```python
from build123d import *

# Parameters (mm, degrees)
CUT_EXTRUDE_START   = 10
CUT_EXTRUDE_1_DEPTH = 112.622366364


with BuildPart() as part:
    # Эскиз1 → Повернуть1 (revolve)
    with BuildSketch(Plane.XY):
        Polygon((0, 0), (0, 12.5), (15, 12.5), (15, 14), (55, 14), (55, 12.5), (70, 12.5), (70, 11), (120, 11), (120, 0), align=None)
    revolve(axis=Axis((120, 0, 0), (-1, 0, 0)))

    # Эскиз3 → Вырез-Вытянуть1 (cut, through all)
    with BuildSketch(Plane(origin=(0, 0, 0), x_dir=(1, 0, 0), z_dir=(0, 1, 0)).offset(CUT_EXTRUDE_START)):
        with BuildLine():
            Line((21, 4), (49, 4))
            ThreePointArc((49, 4), (53, 0), (49, -4))
            Line((49, -4), (21, -4))
            ThreePointArc((21, -4), (17, 0), (21, 4))
        make_face()
    extrude(amount=CUT_EXTRUDE_1_DEPTH, mode=Mode.SUBTRACT)


solid = part.part
```
Verification items for the finished model (mm, model axes). A direction names the side the tool comes from. Round coordinates to 2 decimals unless told otherwise and drop trailing zeros. Write each loop counter-clockwise with the first axis right and the second up, starting at its lowest first coordinate (ties: lowest second). Pieces come first, ordered by that corner, then holes.
1. Section check B-B on z = -1.25. Enter the section's corners in (x, y).
2. Gauge pin test, flat ends, axial feed: P1, Ø12, axis at x = 34.5, y = -8.5, coming from the -Z side (3 decimals); P2, Ø2, axis at x = 60.5, z = -2, coming from the -Y side; P3, Ø5, axis at y = 6.5, z = 2.5, coming from the -X side; P4, Ø2, axis at x = 40.5, y = 7.5, coming from the -Z side. Record the tip position at first contact, or that the pin passes through.
3. Section check D-D on y = -7.75. Enter the section's corners in (x, z).
4. Scan lines: L1, parallel to X at y = 9, z = 7; L2, parallel to Z at x = 46.5, y = 0.5; L3, parallel to Y at x = 53.5, z = -4.25. Record each from-to range of solid material in increasing order.
5. Section check C-C on x = 86. Enter the section's corners in (y, z), plus the area to 3 significant figures.
6. Access from +Z, -Z, +X, -X, +Y, -Y to the whole of each face (thin tool, end or side, straight path). Record for faces 4 (the cylindrical face through (62.605, 11.923, -3.755)), 5 (the flat face through (15, 5.3, -11.5)), 6 (the flat face through (35, 12, 4)).
7. Draft check along Z on faces 1 (the cylindrical face through (35.28, 12.932, 5.362)), 2 (the cylindrical face through (53, 12, 0)), 3 (the flat face through (70, 5, 10)). Enter one of: +Z half, -Z half, draft (parallel to the pull), parting line (faces both ways), or undercut.
8. Section check A-A on y = 0. Enter the section's corners in (x, z), plus the area to 3 significant figures.
Answer:
1. outline: (0, -12.44) - (15, -12.44) - (15, -13.94) - (55, -13.94) - (55, -12.44) - (70, -12.44) - (70, -10.93) - (120, -10.93) - (120, 10.93) - (70, 10.93) - (70, 12.44) - (55, 12.44) - (55, 13.94) - (52.8, 13.94) - (52.8, 10) - (17.2, 10) - (17.2, 13.94) - (15, 13.94) - (15, 12.44) - (0, 12.44) - close
2. P1: stops at z = -13.775
2. P2: stops at y = -12.46
2. P3: stops at x = 0
2. P4: stops at z = -12.4
3. outline: (0, -9.81) - (15, -9.81) - (15, -11.66) - (55, -11.66) - (55, -9.81) - (70, -9.81) - (70, -7.81) - (120, -7.81) - (120, 7.81) - (70, 7.81) - (70, 9.81) - (55, 9.81) - (55, 11.66) - (15, 11.66) - (15, 9.81) - (0, 9.81) - close
4. L1: x = 0 to 70
4. L2: z = -13.99 to 13.99
4. L3: y = -13.34 to 13.34
5. outline: circle Ø22 at (0, 0)
5. area: 380 mm2
6. face 4: +X
6. face 5: -X
6. face 6: +Y
7. face 1: parting line
7. face 2: undercut
7. face 3: draft
8. outline: (0, -12.5) - (15, -12.5) - (15, -14) - (55, -14) - (55, -12.5) - (70, -12.5) - (70, -11) - (120, -11) - (120, 11) - (70, 11) - (70, 12.5) - (55, 12.5) - (55, 14) - (15, 14) - (15, 12.5) - (0, 12.5) - close
8. area: 2,970 mm2
